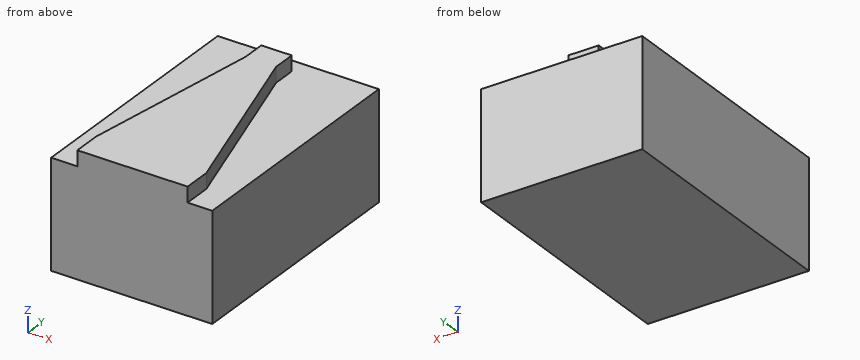
from build123d import *

# Parameters (mm, degrees)
F0_W       = 128.8954913616
F0_H       = 86.3029435277
F1_DEPTH   = 198.374
F2_W       = 88.2518328726
F2_H       = 22.2966937294
F2_W_2     = 24.353325367
F2_H_2     = 18.542567268
F3_DEPTH   = 12.192
F3_FACE_W  = 24.353325367
F3_FACE_H  = 12.192
F3_FACE1_W = 88.2518328726
F3_FACE1_H = 12.192


with BuildPart() as f1:
    # F0 (on Front) → F1 (new body)
    with BuildSketch(Plane.XZ):
        with Locations((64.4477456808, 43.1514717638)):
            Rectangle(F0_W, F0_H)
    extrude(amount=F1_DEPTH)

    # F2 (on face) → F3 (join)
    with BuildSketch(Plane.XY.offset(86.3029435277)):
        with Locations((65.0349687785, -187.2256531353)):
            Rectangle(F2_W, F2_H)
        with Locations((55.3243383765, -21.625594236)):
            Rectangle(F2_W_2, F2_H_2)
    extrude(amount=F3_DEPTH)

    # F3_face (on face) → F4 section 0
    with BuildSketch(Plane(origin=(55.3243383765, -30.89687787, 92.3989435277), x_dir=(1, 0, 0), z_dir=(0, -1, 0))):
        Rectangle(F3_FACE_W, F3_FACE_H)
    # F3_face1 (on face) → F4 section 1
    with BuildSketch(Plane(origin=(65.0349687785, -176.0773062706, 92.3989435277), x_dir=(-1, 0, 0), z_dir=(0, 1, 0))):
        Rectangle(F3_FACE1_W, F3_FACE1_H)
    loft()


solid = f1.part
Geometry check sheet. Reference: the model listing, model coordinates, mm. Round coordinates to 2 decimals unless told otherwise and drop trailing zeros. Loops run counter-clockwise (first coordinate to the right, second up) from the corner with the lowest first, then second, coordinate; pieces in that order, holes last. Notation, with made-up numbers: (-3.75, -33.75) -> (14.25, -33.75) arc R20 cw to (14.25, -4.75) -> close; hole circle Ø9 at (-26, 77). An arc over 180 degrees is marked (long way). Answer as a JSON object with one key per item and string values. Group by question number.
Item 1: Thickness scan on line 1 along Z through (x, y) = (35, -73); line 2 along X through (y, z) = (-166, 94). Record the ranges inside material, lowest first.
Item 2: Depth check by flat-ended pin: pin 1 Ø3.5 at (y, z) = (-190, 95) entering from -X; pin 2 Ø3.5 at (x, z) = (52.5, 93) entering from +Y; pin 3 Ø10 at (y, z) = (-186.5, 93.5) entering from +X. Enter the tip coordinate at first touch or a pass-through.
Item 3: Cross-section at B-B, the plane x = 103. Record the cut outline in (y, z).
Item 4: Cross-section at D-D, the plane x = 11.5. Record the cut outline in (y, z), plus the area to 3 significant figures.
Item 5: Cross-section at C-C, the plane y = -161. Record the cut outline in (x, z), plus the area to 3 significant figures.
Item 6: Cross-section at A-A, the plane y = -18.5. Record the cut outline in (x, z), plus the area to 3 significant figures.
Determined:
{
 "1": {"line 1": "z = 0 to 86.3", "line 2": "x = 22.45 to 106.27"},
 "2": {"pin 1": "stops at x = 20.91", "pin 2": "stops at y = -12.35", "pin 3": "stops at x = 109.16"},
 "3": {"outline": "(-198.37, 0) -> (0, 0) -> (0, 86.3) -> (-154.61, 86.3) -> (-154.61, 98.49) -> (-198.37, 98.49) -> close"},
 "4": {"outline": "(-198.37, 0) -> (0, 0) -> (0, 86.3) -> (-198.37, 86.3) -> close", "area": "17,100 mm²"},
 "5": {"outline": "(0, 0) -> (128.9, 0) -> (128.9, 86.3) -> (104.83, 86.3) -> (104.83, 98.49) -> (23.22, 98.49) -> (23.22, 86.3) -> (0, 86.3) -> close", "area": "12,100 mm²"},
 "6": {"outline": "(0, 0) -> (128.9, 0) -> (128.9, 86.3) -> (67.5, 86.3) -> (67.5, 98.49) -> (43.15, 98.49) -> (43.15, 86.3) -> (0, 86.3) -> close", "area": "11,400 mm²"}
}
